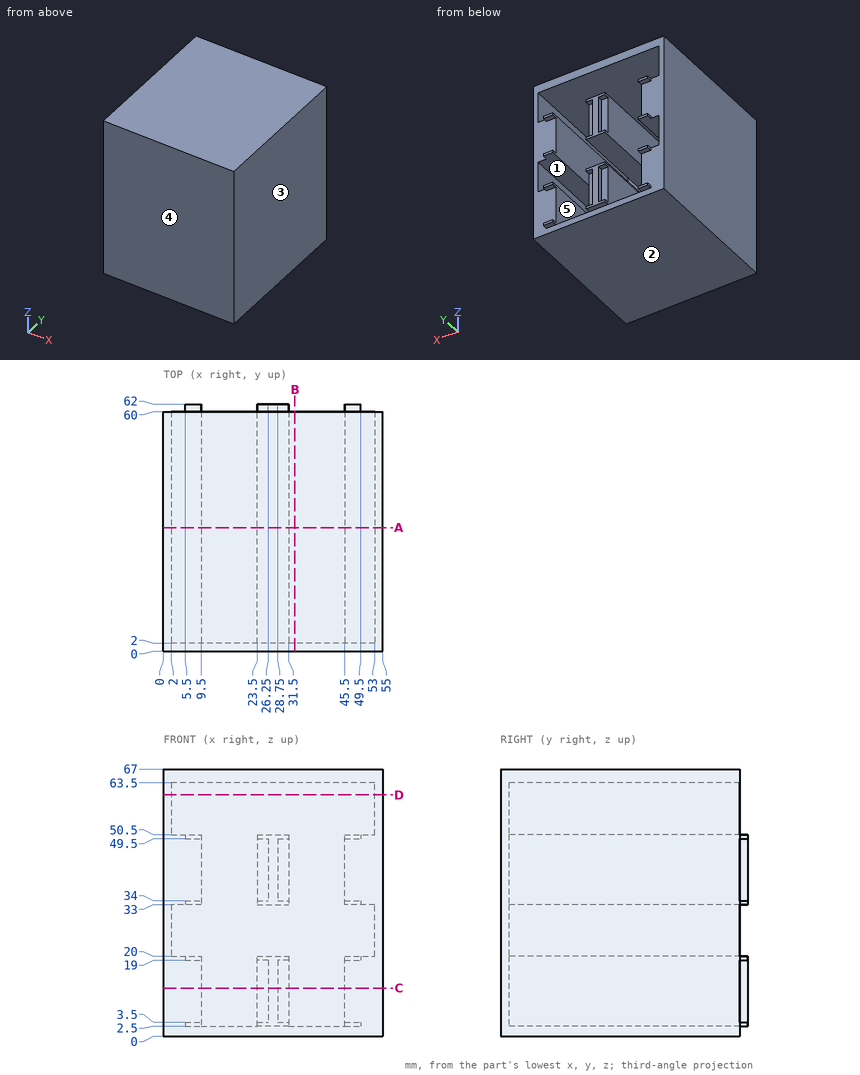
For this review, use the dimensioned drawing (mm, ordinates from the lowest corner) and the shaded views. A direction names the side the tool comes from. Coordinates: 2 decimals unless noted, no trailing zeros. Loops run counter-clockwise (first coordinate to the right, second up) from the corner with the lowest first, then second, coordinate; pieces in that order, holes last.
1. For line 1 (Z direction, x = 50.5, y = 4); line 2 (X direction, y = 55.5, z = 10); line 3 (Z direction, x = 20.5, y = 8), list the stretches that pass through material, from the lowest coordinate up.
2. Mouldability with a two-part tool opening along Z and no side actions: class the marked faces 1, 2 and 3 as +Z half, -Z half, draft (parallel to the pull), parting line (faces both ways), or undercut.
3. For the marked faces 4 and 5, list the 3-axis set-ups (+Z, -Z, +X, -X, +Y, -Y) from which the entire face can be reached by the end or side of a thin tool; tool diameter is ignored.
4. Add section C-C, the plane z = 12. Give the boundary of the cut face in (x, y).
5. Add section D-D, the plane z = 60.5. Give the boundary of the cut face in (x, y), then the cut area to 3 significant figures.
6. Add section B-B, the plane x = 33. Give the boundary of the cut face in (y, z).
7. Add section A-A, the plane y = 31. Give the boundary of the cut face in (x, z).
8. Insertion check: P1, Ø0.6, axis at x = 24.5, y = 60.5, coming from the +Z side; P2, Ø0.8, axis at x = 31, z = 11, coming from the +Y side; P3, Ø2, axis at y = 61.5, z = 7.5, coming from the +X side. Each pin has a flat end and moves straight along its axis. Give the tip position at first contact, or say it passes through.
Result:
1. line 1: z = 0 to 20, 33 to 50.5, 63.5 to 67
1. line 2: x = 0 to 9.5, 23.5 to 31.5, 45.5 to 55
1. line 3: z = 0 to 2.5, 63.5 to 67
2. face 1: undercut
2. face 2: -Z half
2. face 3: draft
3. face 4: +Z, -Z, +X, -X, -Y
3. face 5: +Y
4. outline: (0, 0) - (55, 0) - (55, 60) - (45.5, 60) - (45.5, 2) - (31.5, 2) - (31.5, 60) - (28.75, 60) - (28.75, 62) - (26.25, 62) - (26.25, 60) - (23.5, 60) - (23.5, 2) - (9.5, 2) - (9.5, 60) - (0, 60) - close
5. outline: (0, 0) - (55, 0) - (55, 60) - (53, 60) - (53, 2) - (2, 2) - (2, 60) - (0, 60) - close
5. area: 342 mm2
6. outline: (0, 0) - (60, 0) - (60, 2.5) - (2, 2.5) - (2, 63.5) - (60, 63.5) - (60, 67) - (0, 67) - close
7. outline: (0, 0) - (55, 0) - (55, 67) - (0, 67) - close; (23.5, 33) - (31.5, 33) - (31.5, 50.5) - (23.5, 50.5) - close; hole (2, 20) - (9.5, 20) - (9.5, 2.5) - (23.5, 2.5) - (23.5, 20) - (31.5, 20) - (31.5, 2.5) - (45.5, 2.5) - (45.5, 20) - (53, 20) - (53, 33) - (45.5, 33) - (45.5, 50.5) - (53, 50.5) - (53, 63.5) - (2, 63.5) - (2, 50.5) - (9.5, 50.5) - (9.5, 33) - (2, 33) - close
8. P1: stops at z = 50.5
8. P2: stops at y = 60
8. P3: stops at x = 28.75
